```python
from build123d import *

# Parameters (mm, degrees)
CONG_1_R = 1.1


with BuildPart() as part:
    # Esquisse2 → Base-Révolution (revolve)
    with BuildSketch(Plane.XY, mode=Mode.PRIVATE) as base_r_volution_sk:
        Polygon((39.85, 4.542160182), (33.85, 5.600122066), (33.85, 8.75), (38.85, 8.75), (38.85, 12), (41.85, 12), (41.85, 7), (39.85, 7), align=None)
    revolve(base_r_volution_sk.sketch.rotate(Axis((0, 0, 0), (1, 0, 0)), 90), axis=Axis((0, 0, 0), (1, 0, 0)))

    # Congé1
    cong_1_edges = [part.edges().sort_by_distance(p)[0] for p in [
        (38.85, 0, -8.75),
        (38.85, 0, -12),
    ]]
    fillet(cong_1_edges, radius=CONG_1_R)


solid = part.part
```
Read the model definition and answer for the solid it produces. Units are mm, in the model's axes. A direction names the side the tool comes from. Give positions to 0.01 mm unless a question says otherwise; leave off trailing zeros. Order: outer loops, then holes, each group sorted by start corner. A loop starts at its lowest first (then second) coordinate and runs counter-clockwise, first axis right, second up.
(1) Straight lines are drawn through the part: L1, parallel to Y at x = 40.95, z = 0; L2, parallel to Y at x = 35.75, z = -1.25; L3, parallel to Z at x = 38.5, y = -1. For each, find the intervals that lie inside material, in ascending order.
(2) Given pin 1 (2 mm diameter, centred on x = 35, z = 7, fed in from +Y); pin 2 (1.5 mm diameter, centred on x = 36, z = 0.5, fed in from -Y); pin 3 (3 mm diameter, centred on x = 39, z = 5, fed in from +Y), each flat-ended and moving along its own axis, determine where each tip first touches the part or whether it passes through.
(3) Find section D-D (x = 38.5). Give the vertices of the cut face in (y, z).
(4) For faces 4 (the flat face through (41.85, 5.2, 5.2)), 5 (the cylindrical face through (40.84, 6.21, 3.23)), 6 (the flat face through (38.85, 6, 8)), determine the directions among +Z, -Z, +X, -X, +Y, -Y from which every point of the face is accessible in a straight line to the end or side of a thin tool.
(5) Find section A-A (z = 0). Give the vertices of the cut face in (x, y).
(6) Find section C-C (x = 40.5). Give the vertices of the cut face in (y, z), plus the area to 3 significant figures.
(7) For a pull along Y with two mould halves and no side action, classify faces 1 (the flat face through (33.85, 6, 0)), 2 (the cylindrical face through (40.913, -3.604, 11.446)), 3 (the flat face through (39.85, 5, 0)) as released by +Y, released by -Y, zero draft, split by the parting line, or undercut.
Result sheet:
1. L1: y = -12 to -7, 7 to 12
1. L2: y = -8.66 to -5.11, 5.11 to 8.66
1. L3: z = -8.99 to -4.67, 4.67 to 8.99
2. pin 1: stops at y = 6.37
2. pin 2: stops at y = -8.75
2. pin 3: stops at y = 11.4
3. outline: circle Ø18.09 at (0, 0); hole circle Ø9.56 at (0, 0)
4. face 4: +Z, -Z, +X, +Y, -Y
4. face 5: +X
4. face 6: -X
5. outline: (33.85, -8.75) - (37.75, -8.75) arc R1.1 cw to (38.85, -9.85) - (38.85, -10.9) arc R1.1 ccw to (39.95, -12) - (41.85, -12) - (41.85, -7) - (39.85, -7) - (39.85, -4.54) - (33.85, -5.6) - close; (33.85, 5.6) - (39.85, 4.54) - (39.85, 7) - (41.85, 7) - (41.85, 12) - (39.95, 12) arc R1.1 ccw to (38.85, 10.9) - (38.85, 9.85) arc R1.1 cw to (37.75, 8.75) - (33.85, 8.75) - close
6. outline: circle Ø24 at (0, 0); hole circle Ø14 at (0, 0)
6. area: 298 mm2
7. face 1: zero draft
7. face 2: split by the parting line
7. face 3: undercut
